Source: CAD feature listing. Evaluate the final solid. Frame: model axes, mm. Face numbers are marked on the shaded views. A direction names the side the tool comes from. Coordinates: 2 decimals unless noted, no trailing zeros. Write each loop counter-clockwise with the first axis right and the second up, starting at its lowest first coordinate (ties: lowest second). Pieces come first, ordered by that corner, then holes. Notation, with made-up numbers: (88, 33.5) -> (147, 33.5) arc R27 ccw to (147, 66.5) -> close; hole circle Ø11 at (-15.75, 88). An arc over 180 degrees is marked (long way). Write item = value, one per line.
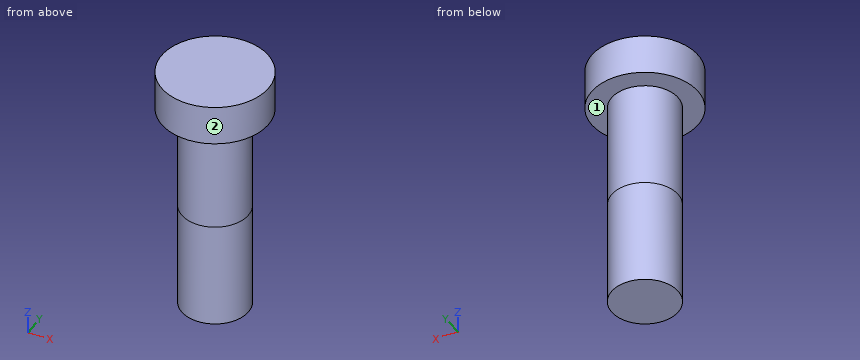
Autodesk Inventor part; units mm, degrees
ref_plane "YZ Plane" through (0, 0, 0) normal (1, 0, 0) x (0, 1, 0)
ref_plane "XZ Plane" through (0, 0, 0) normal (0, 1, 0) x (-1, 0, 0)
ref_plane "XY Plane" through (0, 0, 0) normal (0, 0, 1) x (1, 0, 0)
sketch "Sketch1" plane through (0, 0, 0) normal (0, 0, 1) x (1, 0, 0)
  circle A0 centre (0, 0) radius 1.5875
  dimension "d0" = 3.175
extrude "Extrusion1" add sketch "Sketch1" along normal blind 5.08
sketch "Sketch2" plane through (0, 0, 5.08) normal (0, 0, 1) x (1, 0, 0)
  circle A0 centre (0, 0) radius 2.54
  dimension "d3" = 5.08
extrude "Extrusion2" add sketch "Sketch2" along normal blind 1.905
thread "Thread1"
sketch "Sketch3" plane through (0, 0, 0) normal (0, 0, -1) x (-1, 0, 0)
  circle A0 centre (0, 0) radius 1.5875
extrude "Extrusion3" add sketch "Sketch3" along normal blind 5.08
properties part number "ScrewLong" material "Stainless Steel"
1) Cut plane C-C, the plane z = 6.25. Output: boundary loops of the cut face in (x, y), and give its area (3 significant figures).
Answer block:
outline = circle Ø5.08 at (0, 0)
area = 20.3 mm2
2) Cut plane A-A, the plane x = 0. Output: boundary loops of the cut face in (y, z) (1 decimal), and give its area (3 significant figures).
Answer block:
outline = (-2.5, 5.1) -> (-1.6, 5.1) -> (-1.6, -5.1) -> (1.6, -5.1) -> (1.6, 5.1) -> (2.5, 5.1) -> (2.5, 7) -> (-2.5, 7) -> close
area = 41.9 mm2
3) Reachability of the marked faces 1 and 2 from +Z, -Z, +X, -X, +Y, -Y: full face, straight path, thin tool, end or side. Return the list, or none.
Answer block:
face_1 = -Z
face_2 = +Z, -Z
4) Material intervals for probe 1 along Z at (x, y) = (2.1, 0.35) (3 decimals); probe 2 along Y at (x, z) = (0.25, 3.5); probe 3 along X at (y, z) = (-2.05, 5.5), sorted ascending. Write a range as [from, to].
Answer block:
probe_1 = [5.08, 6.985]
probe_2 = [-1.57, 1.57]
probe_3 = [-1.5, 1.5]
5) First-contact query: pin 1 Ø2 at (x, z) = (0.5, -2) entering from +Y; pin 2 Ø1 at (y, z) = (1, 2) entering from +X; pin 3 Ø1 at (x, z) = (0.5, -1.5) entering from -Y. Flat tips, straight axial feed; report the tip coordinate or a pass-through.
Answer block:
pin_1 = 1.59
pin_2 = 1.51
pin_3 = -1.59
6) Cut plane D-D, the plane z = -2.5. Output: boundary loops of the cut face in (x, y) (1 decimal), and give its area (3 significant figures).
Answer block:
outline = circle Ø3.2 at (0, 0)
area = 7.92 mm2
